The figure shows three views and two pictorial views of one solid part (mm, origin at its lowest corner). Answer the questions. Coordinates: 2 decimals unless noted, no trailing zeros. Order: outer loops, then holes, each group sorted by start corner. A loop starts at its lowest first (then second) coordinate and runs counter-clockwise, first axis right, second up. Notation, with made-up numbers: (81.25, -6.5) - (136.25, -6.5) arc R33 ccw to (136.25, 29.5) - close; hole circle Ø11 at (26, 30.5). An arc over 180 degrees is marked (long way). Use one line per item in the form item = value. Start each with the question number.
Item 1: The mould has two halves that part along X. Classify the marked faces 1, 2 and 3: released by +X, released by -X, zero draft, split by the parting line, or undercut.
Item 2: Consider line 1 along Z through (x, y) = (8.5, 2) (1 decimal); line 2 along X through (y, z) = (21.5, 7); line 3 along Y through (x, z) = (20, 21.5). Determine where each line is inside the solid, lowest interval first. Write a range as [from, to].
Item 3: Section C-C, the plane z = 14 is taken. Write down the section's boundary in (x, y), and give its area (3 significant figures).
Item 4: Each of these flat-tipped pins is pushed along its axis until it touches: pin 1 Ø4 at (x, z) = (28.58, 4.76) entering from +Y; pin 2 Ø1 at (x, z) = (22.5, 23.5) entering from +Y; pin 3 Ø5 at (x, y) = (20.5, 3) entering from +Z (1 decimal). Where does it stop, or does it pass through?
Item 5: Section B-B, the plane y = 33 is taken. Write down the section's boundary in (x, z) (1 decimal).
Item 6: Section D-D, the plane y = 17 is taken. Write down the section's boundary in (x, z) (1 decimal).
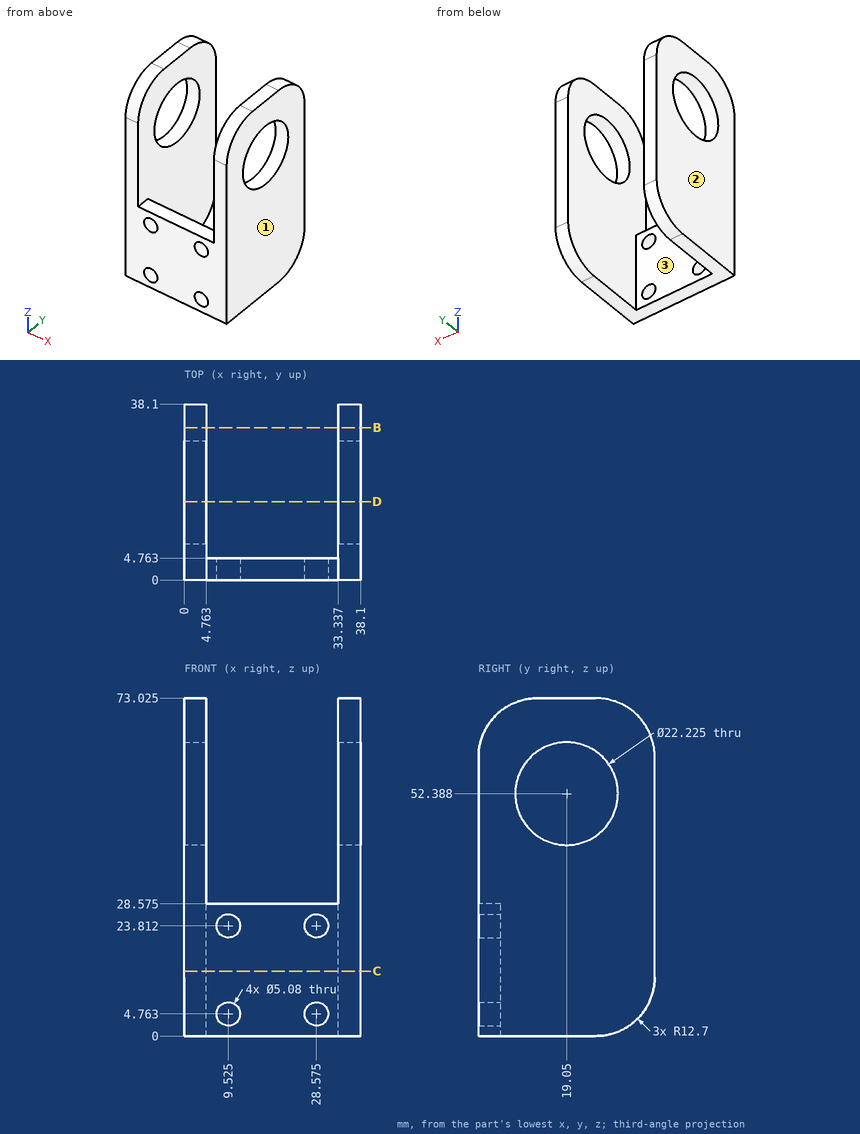
Response:
q1.face_1 = released by +X
q1.face_2 = released by -X
q1.face_3 = undercut
q2.line_1 = [0, 2.4], [7.1, 21.5], [26.1, 28.6]
q2.line_2 = [0, 4.76], [33.34, 38.1]
q2.line_3 = [0, 4.76]
q3.outline = (0, 0) - (38.1, 0) - (38.1, 38.1) - (33.34, 38.1) - (33.34, 4.76) - (4.76, 4.76) - (4.76, 38.1) - (0, 38.1) - close
q3.area = 499 mm2
q4.pin_1 = through
q4.pin_2 = 4.76
q4.pin_3 = 28.6
q5.outline = (0, 2.5) - (4.8, 2.5) - (4.8, 70.5) - (0, 70.5) - close; (33.3, 2.5) - (38.1, 2.5) - (38.1, 70.5) - (33.3, 70.5) - close
q6.outline = (0, 0) - (4.8, 0) - (4.8, 41.5) - (0, 41.5) - close; (0, 63.3) - (4.8, 63.3) - (4.8, 73) - (0, 73) - close; (33.3, 0) - (38.1, 0) - (38.1, 41.5) - (33.3, 41.5) - close; (33.3, 63.3) - (38.1, 63.3) - (38.1, 73) - (33.3, 73) - close
